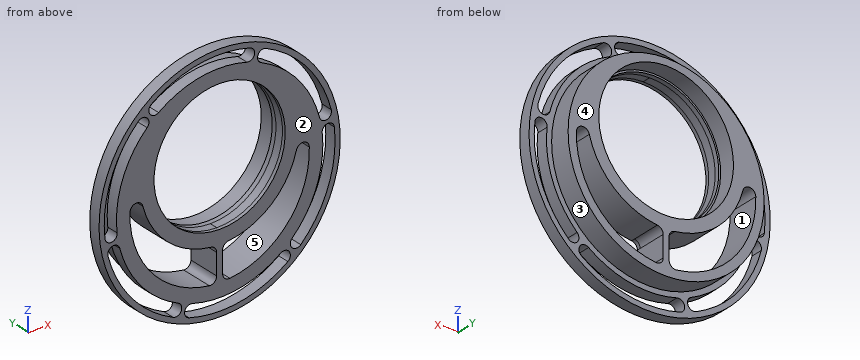
from build123d import *

# Parameters (mm, degrees)
SKETCH1_R               = 61.912499999999994
SKETCH1_R_2             = 35.05199999999999
BOSS_EXTRUDE1_DEPTH     = 4.521199999999999
SKETCH3_R               = 52.38750000000001
BOSS_EXTRUDE2_DEPTH     = 11.43
SKETCH4_R               = 35.05199999999999
CUT_EXTRUDE1_DEPTH      = 89.99862973068743
SKETCH9_R               = 36.000000009
CUT_EXTRUDE3_DEPTH      = 8.889999999999999
CUT_EXTRUDE6_DEPTH      = 4.5212
CIRPATTERN2_COUNT       = 6
CUT_EXTRUDE7_DEPTH      = 89.99862973068743
CUT_EXTRUDE7_DEPTH_BACK = 89.99862973068743
SKETCH28_R              = 61.912499999999994
BOSS_EXTRUDE6_DEPTH     = 1.9049999999999998
SKETCH29_R              = 64.4525
SKETCH29_R_2            = 61.912499999999994
BOSS_EXTRUDE7_DEPTH     = 6.4262


with BuildPart() as part:
    # Sketch1 → Boss-Extrude1 (new body)
    with BuildSketch(Plane(origin=(0, 0, 0), x_dir=(1, 0, 0), z_dir=(0, 1, 0))):
        with Locations(Location((0, 0, 0), (0, 0, 270))):
            Circle(SKETCH1_R)
        with Locations(Location((0, -12.7, 0), (0, 0, 270))):
            Circle(SKETCH1_R_2, mode=Mode.SUBTRACT)
    extrude(amount=BOSS_EXTRUDE1_DEPTH)

    # Sketch3 → Boss-Extrude2 (add)
    with BuildSketch(Plane(origin=(0, 4.521199999999999, 0), x_dir=(1, 0, 0), z_dir=(0, 1, 0))):
        with Locations(Location((0, 0, 0), (0, 0, 270))):
            Circle(SKETCH3_R)
    extrude(amount=BOSS_EXTRUDE2_DEPTH)

    # Sketch4 → Cut-Extrude1 (cut, through all)
    with BuildSketch(Plane.XZ):
        with Locations(Location((0, 12.7, 0), (0, 0, 270))):
            Circle(SKETCH4_R)
    extrude(amount=-CUT_EXTRUDE1_DEPTH, mode=Mode.SUBTRACT)

    # Sketch9 → Cut-Extrude3 (cut)
    with BuildSketch(Plane(origin=(0, 15.951199999999998, 0), x_dir=(1, 0, 0), z_dir=(0, 1, 0))):
        with Locations(Location((0, -12.7, 0), (0, 0, 270))):
            Circle(SKETCH9_R)
    extrude(amount=-CUT_EXTRUDE3_DEPTH, mode=Mode.SUBTRACT)

    # Sketch26 → Cut-Extrude6 (cut)
    with BuildSketch(Plane(origin=(0, 4.521199999999999, 0), x_dir=(1, 0, 0), z_dir=(0, 1, 0))):
        with BuildLine():
            ThreePointArc((-61.31569012651589, 6.729759543927394), (-58.13186307655321, -20.629833117571987), (-43.356751785354874, -43.87591131626929))
            ThreePointArc((-43.356751785354874, -43.87591131626929), (-38.740981882715914, -43.84844086137017), (-38.76845233761503, -39.23267095873121))
            ThreePointArc((-38.76845233761503, -39.23267095873121), (-51.979963216279714, -18.446647154542955), (-54.82685654096325, 6.017571690194909))
            ThreePointArc((-54.82685654096325, 6.017571690194909), (-57.71517940687332, 9.618082409837466), (-61.31569012651589, 6.729759543927394))
        make_face()
    cut_extrude6 = extrude(amount=-CUT_EXTRUDE6_DEPTH, mode=Mode.SUBTRACT)

    # CirPattern2: Cut-Extrude6 ×6 about axis
    cirpattern2_axis = Axis((1.126e-14, 0, 2.9e-14), (0, 1, 0))
    for i in range(1, CIRPATTERN2_COUNT):
        add(cut_extrude6.rotate(cirpattern2_axis, i * 360 / CIRPATTERN2_COUNT), mode=Mode.SUBTRACT)

    # Sketch27 → Cut-Extrude7 (cut, two sides: drawn at the far end of the back side and taken through both)
    with BuildSketch(Plane(origin=(0, 15.951199999999998, 0), x_dir=(1, 0, 0), z_dir=(0, 1, 0)).offset(-CUT_EXTRUDE7_DEPTH_BACK)):
        with BuildLine():
            Line((-1.5874999999999995, 44.15876017281289), (-1.5874999999999981, 32.860162500535104))
            ThreePointArc((-1.5874999999999981, 32.860162500535104), (-2.4771920261720077, 30.53144033991194), (-4.692981403795235, 29.38917231671267))
            ThreePointArc((-4.692981403795235, 29.38917231671267), (-27.80971442943092, 19.239666311904415), (-41.043217293560936, -2.2608039123771086))
            ThreePointArc((-41.043217293560936, -2.2608039123771086), (-44.807125891813406, -4.871764870752282), (-47.91871765916517, -1.509902033647368))
            ThreePointArc((-47.91871765916517, -1.509902033647368), (-36.283267418970276, 31.337003871676934), (-5.479142857142855, 47.62837704353388))
            ThreePointArc((-5.479142857142855, 47.62837704353388), (-2.7558281236719524, 46.76563211813081), (-1.5874999999999995, 44.15876017281289))
        make_face()
        with BuildLine():
            Line((1.5874999999999995, 44.15876017281289), (1.5874999999999981, 32.860162500535104))
            ThreePointArc((1.5874999999999981, 32.860162500535104), (2.4771920261720073, 30.53144033991194), (4.692981403795235, 29.38917231671267))
            ThreePointArc((4.692981403795235, 29.38917231671267), (27.809714429430915, 19.23966631190442), (41.043217293560936, -2.2608039123771086))
            ThreePointArc((41.043217293560936, -2.2608039123771086), (44.807125891813406, -4.871764870752282), (47.91871765916517, -1.509902033647368))
            ThreePointArc((47.91871765916517, -1.509902033647368), (36.28326741897028, 31.337003871676927), (5.479142857142855, 47.62837704353388))
            ThreePointArc((5.479142857142855, 47.62837704353388), (2.755828123671953, 46.76563211813081), (1.5874999999999995, 44.15876017281289))
        make_face()
    extrude(amount=CUT_EXTRUDE7_DEPTH + CUT_EXTRUDE7_DEPTH_BACK, mode=Mode.SUBTRACT)

    # Sketch28 → Boss-Extrude6 (add)
    with BuildSketch(Plane.XZ):
        with Locations(Location((0, 0, 0), (0, 0, 270))):
            Circle(SKETCH28_R)
        with BuildLine():
            ThreePointArc((-59.67602970675995, -15.610092813558284), (-57.34435464364428, -11.626454047298918), (-53.3607158773849, -13.958129110414555))
            ThreePointArc((-53.3607158773849, -13.958129110414557), (-41.96524665862243, -35.792645055806894), (-22.202058317679402, -50.490236419216366))
            ThreePointArc((-22.202058317679395, -50.490236419216366), (-20.528086000825798, -54.79185275524728), (-24.829702336856723, -56.465825072100834))
            ThreePointArc((-24.82970233685672, -56.465825072100834), (-46.93189109392796, -40.02875363482713), (-59.67602970675995, -15.610092813558284))
        make_face(mode=Mode.SUBTRACT)
        with BuildLine():
            Line((-1.5874999999999986, -32.860162500535104), (-1.5874999999999995, -44.15876017281289))
            ThreePointArc((-1.5874999999999977, -44.15876017281289), (-2.755828123671947, -46.76563211813081), (-5.4791428571428495, -47.62837704353388))
            ThreePointArc((-5.479142857142854, -47.62837704353389), (-36.28326741897027, -31.337003871676924), (-47.918717659165196, 1.5099020336473608))
            ThreePointArc((-47.918717659165196, 1.5099020336473605), (-44.80712589181342, 4.871764870752293), (-41.04321729356092, 2.2608039123771135))
            ThreePointArc((-41.04321729356093, 2.2608039123771135), (-27.8097144294309, -19.239666311904422), (-4.692981403795217, -29.389172316712667))
            ThreePointArc((-4.692981403795219, -29.38917231671267), (-2.4771920261720033, -30.531440339911942), (-1.587499999999999, -32.860162500535104))
        make_face(mode=Mode.SUBTRACT)
        with BuildLine():
            ThreePointArc((-16.319277921405433, -59.48600412982813), (-18.603372760928732, -55.47489490866959), (-14.592263539770187, -53.1908000691463))
            ThreePointArc((-14.592263539770187, -53.19080006914629), (10.014716557657184, -54.239292210350484), (32.62479822328402, -44.47266472902207))
            ThreePointArc((32.62479822328402, -44.47266472902206), (37.18709340604772, -45.173770345410375), (36.48598778965936, -49.73606552817407))
            ThreePointArc((36.48598778965937, -49.73606552817408), (11.199971982625161, -60.6585867523998), (-16.319277921405433, -59.48600412982813))
        make_face(mode=Mode.SUBTRACT)
        with BuildLine():
            Line((1.5874999999999995, -44.15876017281289), (1.5874999999999981, -32.860162500535104))
            ThreePointArc((1.5874999999999986, -32.860162500535104), (2.4771920261720077, -30.53144033991194), (4.692981403795235, -29.38917231671267))
            ThreePointArc((4.692981403795236, -29.389172316712674), (27.80971442943091, -19.239666311904415), (41.043217293560936, 2.260803912377108))
            ThreePointArc((41.043217293560936, 2.2608039123771118), (44.80712589181342, 4.871764870752304), (47.91871765916518, 1.509902033647373))
            ThreePointArc((47.918717659165196, 1.5099020336473767), (36.28326741897028, -31.337003871676927), (5.479142857142865, -47.62837704353388))
            ThreePointArc((5.479142857142865, -47.628377043533874), (2.755828123671944, -46.765632118130824), (1.587499999999999, -44.15876017281289))
        make_face(mode=Mode.SUBTRACT)
        with BuildLine():
            ThreePointArc((43.35675178535485, -43.8759113162693), (38.740981882715914, -43.848440861370165), (38.76845233761502, -39.232670958731234))
            ThreePointArc((38.76845233761502, -39.232670958731234), (51.9799632162797, -18.44664715454299), (54.82685654096326, 6.017571690194891))
            ThreePointArc((54.826856540963256, 6.017571690194889), (57.715179406873325, 9.61808240983748), (61.31569012651589, 6.729759543927382))
            ThreePointArc((61.3156901265159, 6.729759543927382), (58.131863076553195, -20.62983311757202), (43.35675178535486, -43.87591131626931))
        make_face(mode=Mode.SUBTRACT)
        with BuildLine():
            ThreePointArc((-43.356751785354874, 43.87591131626928), (-38.740981882715914, 43.84844086137017), (-38.76845233761503, 39.23267095873121))
            ThreePointArc((-38.76845233761503, 39.23267095873122), (-51.9799632162797, 18.446647154542973), (-54.82685654096326, -6.017571690194876))
            ThreePointArc((-54.826856540963256, -6.01757169019488), (-57.71517940687332, -9.618082409837479), (-61.31569012651589, -6.729759543927381))
            ThreePointArc((-61.31569012651589, -6.729759543927381), (-58.1318630765532, 20.629833117572), (-43.356751785354874, 43.875911316269274))
        make_face(mode=Mode.SUBTRACT)
        with BuildLine():
            ThreePointArc((16.31927792140503, 59.486004129828245), (18.603372760928355, 55.47489490866972), (14.592263539769828, 53.1908000691464))
            ThreePointArc((14.592263539769828, 53.1908000691464), (-10.014716557657586, 54.23929221035041), (-32.624798223284365, 44.472664729021815))
            ThreePointArc((-32.62479822328437, 44.472664729021815), (-37.187093406048064, 45.17377034541014), (-36.48598778965972, 49.73606552817383))
            ThreePointArc((-36.48598778965972, 49.73606552817383), (-11.19997198262558, 60.65858675239972), (16.31927792140503, 59.48600412982824))
        make_face(mode=Mode.SUBTRACT)
        with BuildLine():
            ThreePointArc((-1.342e-14, 47.75199999999998), (24.785506894150842, 37.48550689415085), (35.05199999999998, 12.7))
            ThreePointArc((35.05199999999998, 12.69999999999999), (24.785506894150842, -12.085506894150853), (-6.44e-15, -22.35199999999998))
            ThreePointArc((-6.44e-15, -22.35199999999998), (-35.05199999999998, 12.700000000000003), (-1.342e-14, 47.75199999999998))
        make_face(mode=Mode.SUBTRACT)
        with BuildLine():
            ThreePointArc((59.676029706759834, 15.61009281355871), (57.344354643644195, 11.626454047299315), (53.3607158773848, 13.958129110414966))
            ThreePointArc((53.3607158773848, 13.958129110414966), (41.96524665862217, 35.79264505580721), (22.20205831767902, 50.49023641921653))
            ThreePointArc((22.20205831767902, 50.49023641921653), (20.528086000825407, 54.79185275524743), (24.829702336856318, 56.465825072101026))
            ThreePointArc((24.829702336856318, 56.46582507210103), (46.931891093927675, 40.02875363482747), (59.676029706759834, 15.610092813558712))
        make_face(mode=Mode.SUBTRACT)
    extrude(amount=BOSS_EXTRUDE6_DEPTH)

    # Sketch29 → Boss-Extrude7 (add, through all)
    with BuildSketch(Plane(origin=(0, 4.521199999999999, 0), x_dir=(1, 0, 0), z_dir=(0, 1, 0))):
        with Locations(Location((0, 0, 0), (0, 0, 270))):
            Circle(SKETCH29_R)
        Circle(SKETCH29_R_2, mode=Mode.SUBTRACT)
    extrude(amount=-BOSS_EXTRUDE7_DEPTH)


solid = part.part
Part model, mm, in its own coordinate system. Face numbers are marked on the shaded views. A direction names the side the tool comes from. Round coordinates to 2 decimals unless told otherwise and drop trailing zeros. Write each loop counter-clockwise with the first axis right and the second up, starting at its lowest first coordinate (ties: lowest second). Pieces come first, ordered by that corner, then holes. Notation, with made-up numbers: M 87.25,69 L 130.25,69 A24 cw 130.25,88 Z; hole C 44,18 d2. An arc over 180 degrees is marked long. Return JSON: item names as keys, results as strings. Group by question number.
(1) Drill centre lines: probe 1 along Z at (x, y) = (27.5, 7); probe 2 along Z at (x, y) = (20, 5.75); probe 3 along Y at (x, z) = (-35.5, 16) (3 decimals). Where is each one in solid material? Low to high.
(2) Saw through at B-B on z = 25.5. Write the cut outline in (x, y) (3 decimals), then the cut area to 3 significant figures.
(3) Pin check, flat tips, straight feed: pin 1 Ø1 at (x, y) = (-31, 12) entering from +Z; pin 2 Ø4 at (x, y) = (30, 4) entering from -Z; pin 3 Ø8 at (y, z) = (1.5, 51) entering from +X. Stop position of each tip, or through.
(4) Saw through at D-D on x = 11. Write the cut outline in (y, z) (3 decimals).
(5) Saw through at A-A on y = 10. Count the separate pieces of the cut face and the enclosed holes in it, then the cut area to 3 significant figures.
(6) Two-plate mould, pull along X, no slides. Class the marked faces 3, 4 and 5: +X half, -X half, draft (parallel to the pull), parting line (faces both ways), or undercut.
(7) Which spindle directions (+Z, -Z, +X, -X, +Y, -Y) get a long thin tool onto all of the face, cutting with end or side? Do the marked faces 1 and 2. Say none if no direction does.
Returned:
{
 "1": {"probe 1": "-44.59 to -39.27, -19.51 to -9.03, 34.43 to 44.59", "probe 2": "-48.42 to -43.57, -24.63 to -16.09, 41.49 to 48.42", "probe 3": "-1.905 to 7.061"},
 "2": {"outline": "M -59.194,-1.905 L -56.166,-1.905 L -56.166,4.521 L -59.194,4.521 Z; M -48.908,-1.905 L -32.631,-1.905 L -32.631,7.061 L -33.648,7.061 L -33.648,15.951 L -45.762,15.951 L -45.762,4.521 L -48.908,4.521 Z; M 32.631,-1.905 L 48.908,-1.905 L 48.908,4.521 L 45.762,4.521 L 45.762,15.951 L 33.648,15.951 L 33.648,7.061 L 32.631,7.061 Z; M 56.166,-1.905 L 59.194,-1.905 L 59.194,4.521 L 56.166,4.521 Z", "area": "530 mm²"},
 "3": {"pin 1": "z = 42.59", "pin 2": "z = -58.05", "pin 3": "x = 44.1"},
 "4": {"outline": "M -1.905,-63.507 L 4.521,-63.507 L 4.521,-60.695 L -1.905,-60.695 Z; M -1.905,-54.048 L 4.521,-54.048 L 4.521,-51.22 L 15.951,-51.22 L 15.951,-46.664 L -1.905,-46.664 Z; M -1.905,-28.196 L 15.951,-28.196 L 15.951,-21.578 L 7.061,-21.578 L 7.061,-20.581 L -1.905,-20.581 Z; M -1.905,45.981 L 7.061,45.981 L 7.061,46.978 L 15.951,46.978 L 15.951,51.22 L 4.521,51.22 L 4.521,54.048 L -1.905,54.048 Z; M -1.905,60.695 L 4.521,60.695 L 4.521,63.507 L -1.905,63.507 Z"},
 "5": {"separate pieces": "1", "enclosed holes": "3", "area": "2,710 mm²"},
 "6": {"face 3": "parting line", "face 4": "draft", "face 5": "undercut"},
 "7": {"face 1": "+Y, -Y", "face 2": "+Z, -Z, +X, -X, -Y"}
}
